For this review, take the finished solid that the model builds, in its own axes (mm). A direction names the side the tool comes from. Coordinates: 2 decimals unless noted, no trailing zeros. One line per item, written item: value. Start each with the question number.
(1) To check wall thickness, follow line 1 along Z through (x, y) = (1.6, 10.5); line 2 along Y through (x, z) = (2.6, 0); line 3 along Z through (x, y) = (-1.4, -2.5). State the ranges of each line that lie inside material, in increasing order.
(2) Mouldability with a two-part tool opening along Z and no side actions: class faces 3 (the flat face through (-3, -3, 11)), 4 (the cylindrical face through (-0.718, -11.429, -36.293)), 5 (the cylindrical face through (0.042, -30.508, -17.357)) as released by +Z, released by -Z, zero draft, split by the parting line, or undercut.
(3) Consider section B-B on y = 0. Count the separate pieces of the cut face and the enclosed holes in it, then the cut area to 3 significant figures.
(4) For faces 1 (the cylindrical face through (0, 0, -15)), 2 (the cylindrical face through (-0.78, 10.39, -4.31)), list the 3-axis set-ups (+Z, -Z, +X, -X, +Y, -Y) from which the entire face can be reached by the end or side of a thin tool; tool diameter is ignored.
(5) Clearance check with flat-ended pins moving along their axes: pin 1 (1 mm diameter, centred on x = 0.5, z = 14, fed in from +Y); pin 2 (11 mm diameter, centred on y = -3.5, z = -3.5, fed in from -X); pin 3 (3 mm diameter, centred on x = 1.5, y = 22.5, fed in from -Z). State where each tip first meets the part, or that it passes through.
```python
from build123d import *

# Parameters (mm, degrees)
CUT_EXTRUDE2_DEPTH      = 58.026485075
FILLET1_R               = 0.5
CUT_EXTRUDE5_DEPTH      = 58.026485145
CUT_EXTRUDE5_DEPTH_BACK = 58.026485145
SKETCH7_R               = 4.2
SKETCH8_R               = 11.25
CUT_EXTRUDE6_DEPTH      = 4.5


with BuildPart() as part:
    # Sketch1 → Revolve2 (revolve)
    with BuildSketch(Plane.XY, mode=Mode.PRIVATE) as revolve2_sk:
        Polygon((-3, 0), (-3, 38.05), (2, 38.05), (2, 40.1), (3, 40.1), (3, 0), align=None)
    revolve(revolve2_sk.sketch.rotate(Axis((3, 0, 0), (-1, 0, 0)), 90), axis=Axis((3, 0, 0), (-1, 0, 0)))

    # Sketch2 → Cut-Extrude2 (cut, through all)
    with BuildSketch(Plane.ZY.offset(-3)):
        with BuildLine():
            Line((14.415571014, 6.656167139), (30.177246505, 15.756174727))
            ThreePointArc((30.177246505, 15.756174727), (30.970527299, 15.84617567), (31.576872502, 15.326810593))
            ThreePointArc((31.576872502, 15.326810593), (35.1, 0), (31.576872502, -15.326810593))
            ThreePointArc((31.576872502, -15.326810593), (30.970527299, -15.84617567), (30.177246505, -15.756174727))
            Line((30.177246505, -15.756174727), (14.415571014, -6.656167139))
            ThreePointArc((14.415571014, -6.656167139), (13.972302174, -6.122171697), (13.983347826, -5.428257877))
            ThreePointArc((13.983347826, -5.428257877), (15, 0), (13.983347826, 5.428257877))
            ThreePointArc((13.983347826, 5.428257877), (13.972302174, 6.122171697), (14.415571014, 6.656167139))
        make_face()
        with BuildLine():
            Line((12.972195341, -9.156167139), (28.733870832, -18.256174727))
            ThreePointArc((28.733870832, -18.256174727), (29.208454332, -18.898175575), (29.061843584, -19.682968463))
            ThreePointArc((29.061843584, -19.682968463), (17.55, -30.397491673), (2.515028919, -35.009779056))
            ThreePointArc((2.515028919, -35.009779056), (1.762072967, -34.744351245), (1.443375673, -34.012349453))
            Line((1.443375673, -34.012349453), (1.443375673, -15.812334278))
            ThreePointArc((1.443375673, -15.812334278), (1.684194871, -15.161454481), (2.290664693, -14.824063386))
            ThreePointArc((2.290664693, -14.824063386), (7.5, -12.990381057), (11.692683133, -9.395805509))
            ThreePointArc((11.692683133, -9.395805509), (12.288107303, -9.039282784), (12.972195341, -9.156167139))
        make_face()
        with BuildLine():
            Line((-1.443375673, -15.812334278), (-1.443375673, -34.012349453))
            ThreePointArc((-1.443375673, -34.012349453), (-1.762072967, -34.744351245), (-2.515028919, -35.009779056))
            ThreePointArc((-2.515028919, -35.009779056), (-17.55, -30.397491673), (-29.061843584, -19.682968463))
            ThreePointArc((-29.061843584, -19.682968463), (-29.208454332, -18.898175575), (-28.733870832, -18.256174727))
            Line((-28.733870832, -18.256174727), (-12.972195341, -9.156167139))
            ThreePointArc((-12.972195341, -9.156167139), (-12.288107303, -9.039282784), (-11.692683133, -9.395805509))
            ThreePointArc((-11.692683133, -9.395805509), (-7.5, -12.990381057), (-2.290664693, -14.824063386))
            ThreePointArc((-2.290664693, -14.824063386), (-1.684194871, -15.161454481), (-1.443375673, -15.812334278))
        make_face()
        with BuildLine():
            Line((-14.415571014, -6.656167139), (-30.177246505, -15.756174727))
            ThreePointArc((-30.177246505, -15.756174727), (-30.970527299, -15.84617567), (-31.576872502, -15.326810593))
            ThreePointArc((-31.576872502, -15.326810593), (-35.1, 0), (-31.576872502, 15.326810593))
            ThreePointArc((-31.576872502, 15.326810593), (-30.970527299, 15.84617567), (-30.177246505, 15.756174727))
            Line((-30.177246505, 15.756174727), (-14.415571014, 6.656167139))
            ThreePointArc((-14.415571014, 6.656167139), (-13.972302174, 6.122171697), (-13.983347826, 5.428257877))
            ThreePointArc((-13.983347826, 5.428257877), (-15, 0), (-13.983347826, -5.428257877))
            ThreePointArc((-13.983347826, -5.428257877), (-13.972302174, -6.122171697), (-14.415571014, -6.656167139))
        make_face()
        with BuildLine():
            Line((-12.972195341, 9.156167139), (-28.733870832, 18.256174727))
            ThreePointArc((-28.733870832, 18.256174727), (-29.208454332, 18.898175575), (-29.061843584, 19.682968463))
            ThreePointArc((-29.061843584, 19.682968463), (-17.55, 30.397491673), (-2.515028919, 35.009779056))
            ThreePointArc((-2.515028919, 35.009779056), (-1.762072967, 34.744351245), (-1.443375673, 34.012349453))
            Line((-1.443375673, 34.012349453), (-1.443375673, 15.812334278))
            ThreePointArc((-1.443375673, 15.812334278), (-1.684194871, 15.161454481), (-2.290664693, 14.824063386))
            ThreePointArc((-2.290664693, 14.824063386), (-7.5, 12.990381057), (-11.692683133, 9.395805509))
            ThreePointArc((-11.692683133, 9.395805509), (-12.288107303, 9.039282784), (-12.972195341, 9.156167139))
        make_face()
        with BuildLine():
            Line((1.443375673, 15.812334278), (1.443375673, 34.012349453))
            ThreePointArc((1.443375673, 34.012349453), (1.762072967, 34.744351245), (2.515028919, 35.009779056))
            ThreePointArc((2.515028919, 35.009779056), (17.55, 30.397491673), (29.061843584, 19.682968463))
            ThreePointArc((29.061843584, 19.682968463), (29.208454332, 18.898175575), (28.733870832, 18.256174727))
            Line((28.733870832, 18.256174727), (12.972195341, 9.156167139))
            ThreePointArc((12.972195341, 9.156167139), (12.288107303, 9.039282784), (11.692683133, 9.395805509))
            ThreePointArc((11.692683133, 9.395805509), (7.5, 12.990381057), (2.290664693, 14.824063386))
            ThreePointArc((2.290664693, 14.824063386), (1.684194871, 15.161454481), (1.443375673, 15.812334278))
        make_face()
    extrude(amount=CUT_EXTRUDE2_DEPTH, mode=Mode.SUBTRACT)

    # Fillet1
    fillet1_edges = [part.edges().sort_by_distance(p)[0] for p in [
        (3, 0, 40.1),
        (2, 0, 40.1),
        (2, 0, 38.05),
    ]]
    fillet(fillet1_edges, radius=FILLET1_R - 0.0001)  # a hair under: the kernel refuses the full size

    # Sketch7 → Cut-Extrude5 (cut, two sides: drawn at the far end of the back side and taken through both)
    with BuildSketch(Plane(origin=(3, 0, 0), x_dir=(0, 0, -1), z_dir=(1, 0, 0)).offset(-CUT_EXTRUDE5_DEPTH_BACK)):
        Circle(SKETCH7_R)
    extrude(amount=CUT_EXTRUDE5_DEPTH + CUT_EXTRUDE5_DEPTH_BACK, mode=Mode.SUBTRACT)

    # Sketch8 → Cut-Extrude6 (cut)
    with BuildSketch(Plane(origin=(-3, 0, 0), x_dir=(0, 0, -1), z_dir=(1, 0, 0))):
        with Locations(Location((0, 0, 0), (0, 0, 90))):
            Circle(SKETCH8_R)
    extrude(amount=CUT_EXTRUDE6_DEPTH, mode=Mode.SUBTRACT)


solid = part.part
```
Geometry check:
1. line 1: z = -36.58 to -33.49, -21.07 to -15.3, -10.71 to 10.71, 15.3 to 21.07, 33.49 to 36.58
1. line 2: y = -40.09 to -4.2, 4.2 to 40.09
1. line 3: z = -37.97 to -35.01, -14.79 to -10.97, 10.97 to 14.79, 35.01 to 37.97
2. face 3: zero draft
2. face 4: split by the parting line
2. face 5: undercut
3. separate pieces: 4
3. enclosed holes: 0
3. area: 106 mm^2
4. face 1: +X, -X
4. face 2: -X
5. pin 1: stops at y = 35.57
5. pin 2: stops at x = 1.5
5. pin 3: stops at z = -33.97
